```python
from build123d import *

# Parameters (mm, degrees)
SKETCH1_W                 = 10
SKETCH1_H                 = 20
CUT_EXTRUDE1_DEPTH        = 13
F_2_0MM_DOWEL_HOLE1_D     = 2
F_2_0MM_DOWEL_HOLE1_DEPTH = 10
F_2_0MM_DOWEL_HOLE1_TIP   = 0.600860619


with BuildPart() as part:
    # Sketch1 → Revolve1 (revolve)
    with BuildSketch(Plane(origin=(0, 0, 0), x_dir=(1, 0, 0), z_dir=(0, 1, 0)), mode=Mode.PRIVATE) as revolve1_sk:
        with Locations((5, 0)):
            Rectangle(SKETCH1_W, SKETCH1_H)
    revolve(revolve1_sk.sketch.rotate(Axis((0, 0, -10), (0, 0, 1)), 180), axis=Axis((0, 0, -10), (0, 0, 1)))

    # Sketch3 → Cut-Extrude1 (cut, symmetric)
    with BuildSketch(Plane(origin=(0, 0, 0), x_dir=(1, 0, 0), z_dir=(0, 1, 0))):
        Polygon((5, -9), (-5, -9), (-2.5, 1), (7.5, 1), align=None)
    extrude(amount=CUT_EXTRUDE1_DEPTH, both=True, mode=Mode.SUBTRACT)

    # Ø2.0mm Dowel Hole1
    with Locations(Plane(origin=(0, 0, -10), x_dir=(-1, 0, 0), z_dir=(0, 0, -1))):
        with Locations((0, 0)):
            Hole(F_2_0MM_DOWEL_HOLE1_D / 2, depth=F_2_0MM_DOWEL_HOLE1_DEPTH)
            with Locations((0, 0, -(F_2_0MM_DOWEL_HOLE1_DEPTH + F_2_0MM_DOWEL_HOLE1_TIP / 2))):  # 118° drill point
                Cone(0, F_2_0MM_DOWEL_HOLE1_D / 2, F_2_0MM_DOWEL_HOLE1_TIP, mode=Mode.SUBTRACT)


solid = part.part
```
The model under review builds one solid part; all positions refer to its coordinate system, in mm. A direction names the side the tool comes from. Round coordinates to 2 decimals unless told otherwise and drop trailing zeros. Loops run counter-clockwise (first coordinate to the right, second up) from the corner with the lowest first, then second, coordinate; pieces in that order, holes last.
Item 1: Take a section at D-D (z = -4). Write out the cut boundary in (x, y).
Determined:
outline: circle Ø20 at (0, 0); hole circle Ø2 at (0, 0)
Item 2: Clearance check with flat-ended pins moving along their axes: pin 1 Ø1.5 at (y, z) = (3, 1.5) entering from +X; pin 2 Ø1.6 at (x, y) = (0, 0) entering from -Z; pin 3 Ø2 at (x, z) = (-6.5, 4) entering from -Y. State where each tip first meets the part, or that it passes through.
Determined:
pin 1: stops at x = 9.74
pin 2: stops at z = 9
pin 3: stops at y = -8.35
Item 3: For faces 1 (the face through (0, -1, -5)), 2 (the face through (2, 0, -1)), 3 (the face through (2, 0, -10)), list the 3-axis set-ups (+Z, -Z, +X, -X, +Y, -Y) from which the entire face can be reached by the end or side of a thin tool; tool diameter is ignored.
Determined:
face 1: -Z
face 2: +Y, -Y
face 3: -Z, +X, -X, +Y, -Y
Item 4: Take a section at B-B (x = 0). Write out the cut boundary in (y, z).
Determined:
outline: (-10, -10) - (-1, -10) - (-1, -1) - (-10, -1) - close; (-10, 9) - (10, 9) - (10, 10) - (-10, 10) - close; (1, -10) - (10, -10) - (10, -1) - (1, -1) - close
Item 5: Take a section at A-A (x = 6). Write out the cut boundary in (y, z).
Determined:
outline: (-8, -10) - (8, -10) - (8, -1) - (-8, -1) - close; (-8, 5) - (8, 5) - (8, 10) - (-8, 10) - close
Item 6: Mouldability with a two-part tool opening along X and no side actions: class faces 4 (the face through (-9.54, -3, -0.14)), 5 (the face through (-3.767, 0.136, 4.07)), 6 (the face through (0, 0, 10)) as released by +X, released by -X, zero draft, split by the parting line, or undercut.
Determined:
face 4: split by the parting line
face 5: undercut
face 6: zero draft
Item 7: Take a section at C-C (y = 3.75). Write out the cut boundary in (x, z).
Determined:
outline: (-9.27, -10) - (9.27, -10) - (9.27, 10) - (-9.27, 10) - close; hole (-5, 9) - (-2.5, -1) - (7.5, -1) - (5, 9) - close
Item 8: For line 1 (Y direction, x = 0, z = -7.5); line 2 (Z direction, x = 4.5, y = -5.5); line 3 (X direction, y = -1, z = 7), list the stretches that pass through material, from the lowest coordinate up.
Determined:
line 1: y = -10 to -1, 1 to 10
line 2: z = -10 to -1, 9 to 10
line 3: x = -9.95 to -4.5, 5.5 to 9.95
